```python
from build123d import *

# Parameters (mm, degrees)
F0_W     = 25.4
F0_H     = 25.4
F1_DEPTH = 50.8
F2_R     = 4.7625
F3_DEPTH = 38.1
F4_W     = 4.7625
F4_H     = 12.7
F5_DEPTH = 12.7


with BuildPart() as f1:
    # F0 (on Top) → F1 (new body)
    with BuildSketch(Plane.XY):
        with Locations((12.7, 12.7)):
            Rectangle(F0_W, F0_H)
    extrude(amount=F1_DEPTH)

    # F2 (on face) → F3 (cut)
    with BuildSketch(Plane.XY.offset(50.8)):
        with Locations((7.9375, 7.9375)):
            Circle(F2_R)
    extrude(amount=-F3_DEPTH, mode=Mode.SUBTRACT)

    # F4 (on face) → F5 (cut)
    with BuildSketch(Plane.YZ.offset(25.4)):
        with Locations((20.47875, 25.4)):
            Rectangle(F4_W, F4_H)
    extrude(amount=-F5_DEPTH, mode=Mode.SUBTRACT)


solid = f1.part
```
Work out the finished part from the listing and answer in its coordinate system (mm). A direction names the side the tool comes from. Round coordinates to 2 decimals unless told otherwise and drop trailing zeros. Loops run counter-clockwise (first coordinate to the right, second up) from the corner with the lowest first, then second, coordinate; pieces in that order, holes last.
(1) The part is cut by section D-D, the plane x = 4.5. Give the vertices of the cut face in (y, z).
Computed values:
outline: (0, 0) - (25.4, 0) - (25.4, 50.8) - (11.23, 50.8) - (11.23, 12.7) - (4.64, 12.7) - (4.64, 50.8) - (0, 50.8) - close
(2) The part is cut by section B-B, the plane z = 26.5. Give the vertices of the cut face in (x, y) (1 decimal).
Computed values:
outline: (0, 0) - (25.4, 0) - (25.4, 18.1) - (12.7, 18.1) - (12.7, 22.9) - (25.4, 22.9) - (25.4, 25.4) - (0, 25.4) - close; hole circle Ø9.5 at (7.9, 7.9)
(3) Each of these flat-tipped pins is pushed along its axis until it touches: P1, Ø1.4, axis at y = 19.5, z = 27, coming from the +X side; P2, Ø3, axis at x = 9.5, y = 7, coming from the +Z side. Where does it stop, or does it pass through?
Computed values:
P1: stops at x = 12.7
P2: stops at z = 12.7
(4) The mould has two halves that part along X. Classify faces 1 (the cylindrical face through (12.48, 9.37, 32.02)), 2 (the flat face through (0, 13, 25)), 3 (the flat face through (13, 13, 50.8)): pulls with the +X half, pulls with the -X half, needs draft (parallel to the pull), parting line crosses it, or undercut.
Computed values:
face 1: undercut
face 2: pulls with the -X half
face 3: needs draft
(5) The part is cut by section A-A, the plane x = 23. Give the vertices of the cut face in (y, z), and give its area (3 significant figures).
Computed values:
outline: (0, 0) - (25.4, 0) - (25.4, 50.8) - (0, 50.8) - close; hole (18.1, 19.05) - (22.86, 19.05) - (22.86, 31.75) - (18.1, 31.75) - close
area: 1,230 mm2
(6) Find the intervals of material crossed by L1, parallel to Y at x = 7.75, z = 34; L2, parallel to Z at x = 23, y = 21.5; L3, parallel to X at y = 5.75, z = 31, in increasing order.
Computed values:
L1: y = 0 to 3.18, 12.7 to 25.4
L2: z = 0 to 19.05, 31.75 to 50.8
L3: x = 0 to 3.71, 12.17 to 25.4
(7) For faces 4 (the flat face through (8, 8, 12.7)), 5 (the flat face through (19, 20, 19.05)), 6 (the flat face through (25.4, 13, 25)), determine the directions among +Z, -Z, +X, -X, +Y, -Y from which every point of the face is accessible in a straight line to the end or side of a thin tool.
Computed values:
face 4: +Z
face 5: +X
face 6: +Z, -Z, +X, +Y, -Y
(8) The part is cut by section C-C, the plane y = 9.75. Give the vertices of the cut face in (x, z).
Computed values:
outline: (0, 0) - (25.4, 0) - (25.4, 50.8) - (12.34, 50.8) - (12.34, 12.7) - (3.53, 12.7) - (3.53, 50.8) - (0, 50.8) - close
